Source: CAD feature listing. Evaluate the final solid. Frame: model axes, mm. Coordinates: 2 decimals unless noted, no trailing zeros. Order: outer loops, then holes, each group sorted by start corner. A loop starts at its lowest first (then second) coordinate and runs counter-clockwise, first axis right, second up. Notation, with made-up numbers: (-16.75, 72) -> (41.25, 72) arc R35 ccw to (41.25, 106) -> close; hole circle Ø1 at (34, 80.25). An arc over 180 degrees is marked (long way). Put each result on its own line as item: value.
from build123d import *

# Parameters (mm, degrees)
F0_R     = 2.75
F1_DEPTH = 1.62


with BuildPart() as f1:
    # F0 (on Top) → F1 (new body)
    with BuildSketch(Plane.XY):
        with BuildLine():
            ThreePointArc((24.405646, -5.418899), (24.850967, -2.725698), (25, 0))
            ThreePointArc((25, 0), (24.709654, 3.799081), (23.845358, 7.509919))
            ThreePointArc((23.845358, 7.509919), (22.884418, 10.06496), (21.650635, 12.5))
            ThreePointArc((21.650635, 12.5), (19.499647, 15.644928), (16.895727, 18.42646))
            ThreePointArc((16.895727, 18.42646), (14.786007, 20.15872), (12.5, 21.650635))
            ThreePointArc((12.5, 21.650635), (9.064726, 23.298728), (5.418899, 24.405646))
            ThreePointArc((5.418899, 24.405646), (2.725698, 24.850967), (0, 25))
            ThreePointArc((0, 25), (-3.799081, 24.709654), (-7.509919, 23.845358))
            ThreePointArc((-7.509919, 23.845358), (-10.06496, 22.884418), (-12.5, 21.650635))
            ThreePointArc((-12.5, 21.650635), (-15.644928, 19.499647), (-18.42646, 16.895727))
            ThreePointArc((-18.42646, 16.895727), (-20.15872, 14.786007), (-21.650635, 12.5))
            ThreePointArc((-21.650635, 12.5), (-23.298728, 9.064726), (-24.405646, 5.418899))
            ThreePointArc((-24.405646, 5.418899), (-24.850967, 2.725698), (-25, 0))
            ThreePointArc((-25, 0), (-24.709654, -3.799081), (-23.845358, -7.509919))
            ThreePointArc((-23.845358, -7.509919), (-22.884418, -10.06496), (-21.650635, -12.5))
            ThreePointArc((-21.650635, -12.5), (-19.499647, -15.644928), (-16.895727, -18.42646))
            ThreePointArc((-16.895727, -18.42646), (-14.786007, -20.15872), (-12.5, -21.650635))
            ThreePointArc((-12.5, -21.650635), (-9.064726, -23.298728), (-5.418899, -24.405646))
            ThreePointArc((-5.418899, -24.405646), (-2.725698, -24.850967), (0, -25))
            ThreePointArc((0, -25), (3.799081, -24.709654), (7.509919, -23.845358))
            ThreePointArc((7.509919, -23.845358), (10.06496, -22.884418), (12.5, -21.650635))
            ThreePointArc((12.5, -21.650635), (15.644928, -19.499647), (18.42646, -16.895727))
            ThreePointArc((18.42646, -16.895727), (20.15872, -14.786007), (21.650635, -12.5))
            ThreePointArc((21.650635, -12.5), (23.298728, -9.064726), (24.405646, -5.418899))
        make_face()
        Circle(F0_R, mode=Mode.SUBTRACT)
        with BuildLine():
            ThreePointArc((-7.509919, 23.845358), (-3.799081, 24.709654), (0, 25))
            Line((0, 25), (1.87548, 29.298078))
            Line((1.87548, 29.298078), (-3.745994, 28.585496))
            Line((-3.745994, 28.585496), (-7.509919, 23.845358))
        make_face()
        with BuildLine():
            ThreePointArc((-18.42646, 16.895727), (-15.644928, 19.499647), (-12.5, 21.650635))
            Line((-12.5, 21.650635), (-13.024826, 26.31062))
            Line((-13.024826, 26.31062), (-17.536874, 22.882769))
            Line((-17.536874, 22.882769), (-18.42646, 16.895727))
        make_face()
        with BuildLine():
            ThreePointArc((-24.405646, 5.418899), (-23.298728, 9.064726), (-21.650635, 12.5))
            Line((-21.650635, 12.5), (-24.43514, 16.273252))
            Line((-24.43514, 16.273252), (-26.628763, 11.048622))
            Line((-26.628763, 11.048622), (-24.405646, 5.418899))
        make_face()
        with BuildLine():
            Line((-28.585496, -3.745994), (-23.845358, -7.509919))
            ThreePointArc((-23.845358, -7.509919), (-24.709654, -3.799081), (-25, 0))
            Line((-25, 0), (-29.298078, 1.87548))
            Line((-29.298078, 1.87548), (-28.585496, -3.745994))
        make_face()
        with BuildLine():
            ThreePointArc((23.845358, 7.509919), (24.709654, 3.799081), (25, 0))
            Line((25, 0), (29.298078, -1.87548))
            Line((29.298078, -1.87548), (28.585496, 3.745994))
            Line((28.585496, 3.745994), (23.845358, 7.509919))
        make_face()
        with BuildLine():
            Line((26.628763, -11.048622), (24.405646, -5.418899))
            ThreePointArc((24.405646, -5.418899), (23.298728, -9.064726), (21.650635, -12.5))
            Line((21.650635, -12.5), (24.43514, -16.273252))
            Line((24.43514, -16.273252), (26.628763, -11.048622))
        make_face()
        with BuildLine():
            Line((-22.882769, -17.536874), (-16.895727, -18.42646))
            ThreePointArc((-16.895727, -18.42646), (-19.499647, -15.644928), (-21.650635, -12.5))
            Line((-21.650635, -12.5), (-26.31062, -13.024826))
            Line((-26.31062, -13.024826), (-22.882769, -17.536874))
        make_face()
        with BuildLine():
            Line((-11.048622, -26.628763), (-5.418899, -24.405646))
            ThreePointArc((-5.418899, -24.405646), (-9.064726, -23.298728), (-12.5, -21.650635))
            Line((-12.5, -21.650635), (-16.273252, -24.43514))
            Line((-16.273252, -24.43514), (-11.048622, -26.628763))
        make_face()
        with BuildLine():
            Line((3.745994, -28.585496), (7.509919, -23.845358))
            ThreePointArc((7.509919, -23.845358), (3.799081, -24.709654), (0, -25))
            Line((0, -25), (-1.87548, -29.298078))
            Line((-1.87548, -29.298078), (3.745994, -28.585496))
        make_face()
        with BuildLine():
            Line((17.536874, -22.882769), (18.42646, -16.895727))
            ThreePointArc((18.42646, -16.895727), (15.644928, -19.499647), (12.5, -21.650635))
            Line((12.5, -21.650635), (13.024826, -26.31062))
            Line((13.024826, -26.31062), (17.536874, -22.882769))
        make_face()
        with BuildLine():
            ThreePointArc((5.418899, 24.405646), (9.064726, 23.298728), (12.5, 21.650635))
            Line((12.5, 21.650635), (16.273252, 24.43514))
            Line((16.273252, 24.43514), (11.048622, 26.628763))
            Line((11.048622, 26.628763), (5.418899, 24.405646))
        make_face()
        with BuildLine():
            ThreePointArc((16.895727, 18.42646), (19.499647, 15.644928), (21.650635, 12.5))
            Line((21.650635, 12.5), (26.31062, 13.024826))
            Line((26.31062, 13.024826), (22.882769, 17.536874))
            Line((22.882769, 17.536874), (16.895727, 18.42646))
        make_face()
    extrude(amount=F1_DEPTH)


solid = f1.part
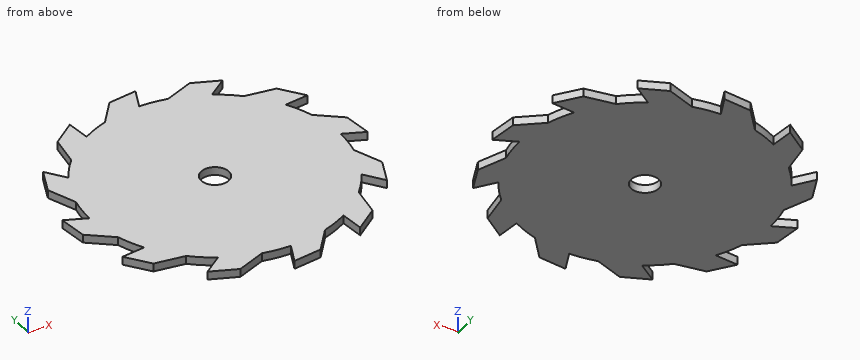
1. Ray query, line 1 along Y through (x, z) = (-1, 0.2); line 2 along Y through (x, z) = (-14.5, 1.25); line 3 along X through (y, z) = (22.5, 1.25). Return the intervals inside material, ascending.
Numbers:
line 1: y = -29.19 to -27.29, -24.98 to -2.56, 2.56 to 28.93
line 2: y = -25.18 to -23.13, -20.37 to 25.19
line 3: x = -17.59 to -12.6, -10.9 to 13.65
2. Cut plane A-A on x = 9.5. Output: boundary loops of the cut face in (y, z).
Numbers:
outline: (-23.12, 0) -> (26.02, 0) -> (26.02, 1.62) -> (-23.12, 1.62) -> close
3. Cut plane B-B on y = -8.5. Output: boundary loops of the cut face in (x, z).
Numbers:
outline: (-23.51, 0) -> (25.62, 0) -> (25.62, 1.62) -> (-23.51, 1.62) -> close
